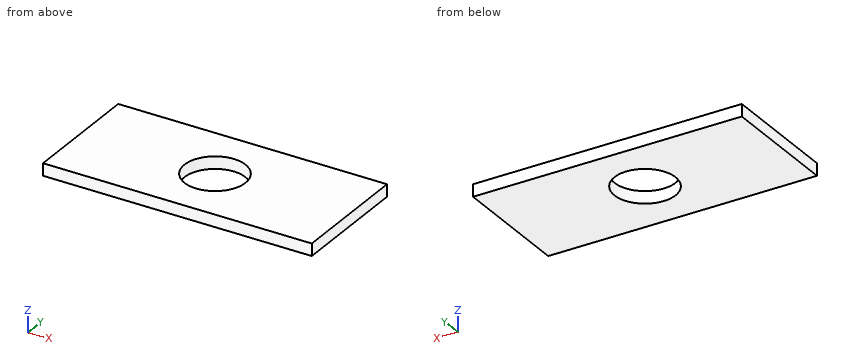
```python
from build123d import *

# Parameters (mm, degrees)
SKETCH1_W           = 11
SKETCH1_H           = 5
SKETCH1_R           = 1.25
BOSS_EXTRUDE1_DEPTH = 0.5
SCALE2_SCALE        = 5


with BuildPart() as part:
    # Sketch1 → Boss-Extrude1 (new body)
    with BuildSketch(Plane.XY):
        with Locations((-44.645074627, 7.944567164)):
            Rectangle(SKETCH1_W, SKETCH1_H)
        with Locations((-44.645074627, 7.944567164)):
            Circle(SKETCH1_R, mode=Mode.SUBTRACT)
    extrude(amount=BOSS_EXTRUDE1_DEPTH)


with BuildPart() as part_1:
    # Scale2: scaled about (0, 0, 0)
    add(part.part.scale(SCALE2_SCALE))


solid = part_1.part
```
Geometry check sheet. Reference: the model listing, model coordinates, mm. Round coordinates to 2 decimals unless told otherwise and drop trailing zeros. Order: outer loops, then holes, each group sorted by start corner. A loop starts at its lowest first (then second) coordinate and runs counter-clockwise, first axis right, second up. Notation, with made-up numbers: (-28.75, 76.25) -> (10.25, 76.25) arc R28 ccw to (10.25, 107.25) -> close; hole circle Ø5 at (44, -3.75). An arc over 180 degrees is marked (long way). Return JSON: item names as keys, results as strings. Group by question number.
Q1. Material ranges on probe 1 along Y at (x, z) = (-223, 1.3); probe 2 along X at (y, z) = (39.5, 1.75); probe 3 along X at (y, z) = (45.25, 1.65), recorded low to high. Write a range as from..to.
Q2. Section check A-A, the plane x = -221. Record the boundary of the cut face in (y, z), plus the area to 3 significant figures.
Q3. Section check C-C, the plane z = 1.5. Record the boundary of the cut face in (x, y), plus the area to 3 significant figures.
Q4. Section check B-B, the plane y = 37. Record the boundary of the cut face in (x, z).
Numbers:
{
 "1": {"probe 1": "27.22..33.48, 45.97..52.22", "probe 2": "-250.73..-229.47, -216.98..-195.73", "probe 3": "-250.73..-226.14, -220.31..-195.73"},
 "2": {"outline": "(27.22, 0) -> (33.88, 0) -> (33.88, 2.5) -> (27.22, 2.5) -> close; (45.56, 0) -> (52.22, 0) -> (52.22, 2.5) -> (45.56, 2.5) -> close", "area": "33.3 mm^2"},
 "3": {"outline": "(-250.73, 27.22) -> (-195.73, 27.22) -> (-195.73, 52.22) -> (-250.73, 52.22) -> close; hole circle Ø12.5 at (-223.23, 39.72)", "area": "1,250 mm^2"},
 "4": {"outline": "(-250.73, 0) -> (-228.85, 0) -> (-228.85, 2.5) -> (-250.73, 2.5) -> close; (-217.6, 0) -> (-195.73, 0) -> (-195.73, 2.5) -> (-217.6, 2.5) -> close"}
}
